The model under review builds one solid part; all positions refer to its coordinate system, in mm. A direction names the side the tool comes from. Give positions to 0.01 mm unless a question says otherwise; leave off trailing zeros. Order: outer loops, then holes, each group sorted by start corner. A loop starts at its lowest first (then second) coordinate and runs counter-clockwise, first axis right, second up.
```python
from build123d import *

# Parameters (mm, degrees)
F0_R     = 12.7
F1_DEPTH = 12.7
F2_W     = 12.7
F2_H     = 50.8
F3_DEPTH = 63.5
F4_R     = 25.39999
F6_D     = 25.4


# Not quite as in the source:
# - a fillet or chamfer is up to 0.001 mm smaller than in the source, because OpenCascade refuses the exact size


with BuildPart() as f1:
    # F0 (on Top) → F1 (new body)
    with BuildSketch(Plane.XY):
        with BuildLine():
            Line((0, 88.9), (0, 0))
            Line((0, 0), (50.8, 0))
            Line((50.8, 0), (50.8, 88.9))
            ThreePointArc((50.8, 88.9), (43.3605122421, 106.8605122421), (25.4, 114.3))
            ThreePointArc((25.4, 114.3), (7.4394877579, 106.8605122421), (0, 88.9))
        make_face()
        with Locations((25.4, 88.9)):
            Circle(F0_R, mode=Mode.SUBTRACT)
    extrude(amount=F1_DEPTH)

    # F2 (on face) → F3 (join)
    with BuildSketch(Plane.XY.offset(12.7)):
        with Locations((6.35, 25.4)):
            Rectangle(F2_W, F2_H)
        with Locations((44.45, 25.4)):
            Rectangle(F2_W, F2_H)
    extrude(amount=F3_DEPTH)

    # F4 (radius 25.4 in the source; OpenCascade refuses exactly that, so slightly less here)
    f4_edges = [f1.edges().sort_by_distance(p)[0] for p in [
        (6.35, 50.8, 76.2),
        (6.35, 0, 76.2),
        (44.45, 0, 76.2),
        (44.45, 50.8, 76.2),
    ]]
    fillet(f4_edges, radius=F4_R)

    # F6 (through all)
    with Locations(Plane(origin=(0, 0, 0), x_dir=(0, -1, 0), z_dir=(-1, 0, 0))):
        with Locations((-25.4, 50.8)):
            Hole(F6_D / 2)


solid = f1.part
```
Item 1: Take a section at B-B (x = 29.5). Give the boundary of the cut face in (y, z), and give its area (3 significant figures).
Values found:
outline: (0, 0) - (76.88, 0) - (76.88, 12.7) - (0, 12.7) - close; (100.92, 0) - (113.97, 0) - (113.97, 12.7) - (100.92, 12.7) - close
area: 1,140 mm2
Item 2: Clearance check with flat-ended pins moving along their axes: pin 1 Ø1.5 at (x, z) = (27.5, 13.5) entering from +Y; pin 2 Ø2 at (x, z) = (11, 55) entering from +Y; pin 3 Ø4 at (x, z) = (14.5, 33) entering from +Y. State where each tip first meets the part, or that it passes through.
Values found:
pin 1: passes through
pin 2: stops at y = 50.6
pin 3: stops at y = 50.8
Item 3: Take a section at A-A (z = 24.5). Give the boundary of the cut face in (x, y), and give its area (3 significant figures).
Values found:
outline: (0, 0) - (12.7, 0) - (12.7, 50.8) - (0, 50.8) - close; (38.1, 0) - (50.8, 0) - (50.8, 50.8) - (38.1, 50.8) - close
area: 1,290 mm2
Item 4: Draft analysis for pull direction Z (two halves, no side actions). For faces 1 (the cylindrical face through (44.5, 15.3, 43.1)), 2 (the cylindrical face through (44.54, 43.56, 68.56)), 3 (the flat face through (12.7, 25, 37)), 4 (the cylindrical face through (6.4, 15.3, 43.1)), state which applies: released by +Z, released by -Z, zero draft, split by the parting line, or undercut.
Values found:
face 1: undercut
face 2: released by +Z
face 3: zero draft
face 4: undercut
Item 5: Take a section at D-D (z = 45.5). Give the boundary of the cut face in (x, y).
Values found:
outline: (0, 0) - (12.7, 0) - (12.7, 13.86) - (0, 13.86) - close; (0, 36.94) - (12.7, 36.94) - (12.7, 50.8) - (0, 50.8) - close; (38.1, 0) - (50.8, 0) - (50.8, 13.86) - (38.1, 13.86) - close; (38.1, 36.94) - (50.8, 36.94) - (50.8, 50.8) - (38.1, 50.8) - close
Item 6: For line 1 (X direction, y = 7.5, z = 30.5); line 2 (Y direction, x = 7, z = 50); line 3 (Y direction, x = 25.4, z = 9), list the stretches that pass through material, from the lowest coordinate up.
Values found:
line 1: x = 0 to 12.7, 38.1 to 50.8
line 2: y = 0 to 12.73, 38.07 to 50.8
line 3: y = 0 to 76.2, 101.6 to 114.3
Item 7: Take a section at C-C (y = 35.5). Give the boundary of the cut face in (x, z), and give its area (3 significant figures).
Values found:
outline: (0, 0) - (50.8, 0) - (50.8, 43.1) - (38.1, 43.1) - (38.1, 12.7) - (12.7, 12.7) - (12.7, 43.1) - (0, 43.1) - close; (0, 58.5) - (12.7, 58.5) - (12.7, 74.11) - (0, 74.11) - close; (38.1, 58.5) - (50.8, 58.5) - (50.8, 74.11) - (38.1, 74.11) - close
area: 1,810 mm2
Item 8: For faces 5 (the flat face through (0, 34, 29)), 6 (the flat face through (25, 58, 12.7)), 7 (the flat face through (38.1, 25, 37)), 8 (the cylindrical face through (23.747, 101.492, 6.261)), 9 (the flat face through (6, 50.8, 31)), list the 3-axis set-ups (+Z, -Z, +X, -X, +Y, -Y) from which the entire face can be reached by the end or side of a thin tool; tool diameter is ignored.
Values found:
face 5: +Z, -Z, -X, +Y, -Y
face 6: +Z, +Y
face 7: +Z, +Y, -Y
face 8: +Z, -Z
face 9: +Z, +X, -X, +Y
